The listing builds one solid part. Answer for the finished solid, in the listing's coordinates (mm). Face numbers are marked on the shaded views. A direction names the side the tool comes from. Coordinates: 2 decimals unless noted, no trailing zeros. Order: outer loops, then holes, each group sorted by start corner. A loop starts at its lowest first (then second) coordinate and runs counter-clockwise, first axis right, second up. Notation, with made-up numbers: (-22.5, 4) -> (27.5, 4) arc R23 cw to (27.5, 22) -> close; hole circle Ø5 at (-15.5, 29). An arc over 180 degrees is marked (long way). Answer in a Markdown table with one row per item. Add a question column.
```python
from build123d import *

# Parameters (mm, degrees)
SKETCH_W     = 25
SKETCH_H     = 32
PAD_DEPTH    = 2
SKETCH001_W  = 22
SKETCH001_H  = 30
PAD001_DEPTH = 16.200001
SKETCH002_W  = 17.2
SKETCH002_H  = 24.2
POCKET_DEPTH = 16
SKETCH003_W  = 1
SKETCH003_H  = 8
PAD002_DEPTH = 10
PAD003_DEPTH = 8.5
FILLET_R     = 1
FILLET001_R  = 0.75
FILLET002_R  = 1
FILLET003_R  = 0.75


with BuildPart() as part:
    # Sketch → Pad (new body)
    with BuildSketch(Plane.XY):
        Rectangle(SKETCH_W, SKETCH_H)
    extrude(amount=PAD_DEPTH)

    # Sketch001 → Pad001 (new body)
    with BuildSketch(Plane(origin=(0, 0, 0), x_dir=(1, 0, 0), z_dir=(0, 0, -1))):
        Rectangle(SKETCH001_W, SKETCH001_H)
    extrude(amount=PAD001_DEPTH)

    # Sketch002 → Pocket (cut)
    with BuildSketch(Plane.XY.offset(2)):
        Rectangle(SKETCH002_W, SKETCH002_H)
    extrude(amount=-POCKET_DEPTH, mode=Mode.SUBTRACT)

    # Sketch003 → Pad002 (new body)
    with BuildSketch(Plane.XY.offset(-14)):
        with Locations((-0.5, 0)):
            Rectangle(SKETCH003_W, SKETCH003_H)
    extrude(amount=PAD002_DEPTH)

    # Sketch004 → Pad003 (new body, symmetric)
    with BuildSketch(Plane.YZ):
        with BuildLine():
            Line((-1.421224, -2.628412), (0.611463, -8.650596))
            ThreePointArc((0.611463, -8.650596), (2.512397, -9.59211), (3.453911, -7.691175))
            Line((3.453911, -7.691175), (1.421224, -1.668991))
            Line((1.421224, -1.668991), (11.362733, 1.686598))
            ThreePointArc((11.362733, 1.686598), (8.973628, 5.807128), (5.169008, 8.672693))
            ThreePointArc((-10.669687, 3.326607), (-1.936582, 3.588753), (5.169008, 8.672693))
            ThreePointArc((-10.669687, 3.326607), (-11.959462, -1.258485), (-11.362733, -5.984001))
            Line((-1.421224, -2.628412), (-11.362733, -5.984001))
        make_face()
    extrude(amount=PAD003_DEPTH, both=True)

    # Fillet
    fillet_edges = [part.edges().sort_by_distance(p)[0] for p in [
        (-12.5, -16, 1),
        (12.5, -16, 1),
        (12.5, 16, 1),
        (-12.5, 16, 1),
    ]]
    fillet(fillet_edges, radius=FILLET_R)

    # Fillet001
    fillet001_edges = [part.edges().sort_by_distance(p)[0] for p in [
        (0, -16, 2),
    ]]
    fillet(fillet001_edges, radius=FILLET001_R)

    # Fillet002
    fillet002_edges = [part.edges().sort_by_distance(p)[0] for p in [
        (0, -10.669687, 3.326607),
        (0, 5.169008, 8.672693),
    ]]
    fillet(fillet002_edges, radius=FILLET002_R)

    # Fillet003
    fillet003_edges = [part.edges().sort_by_distance(p)[0] for p in [
        (8.5, -1.936582, 3.588753),
        (-8.5, -1.936582, 3.588753),
    ]]
    fillet(fillet003_edges, radius=FILLET003_R)


solid = part.part
```
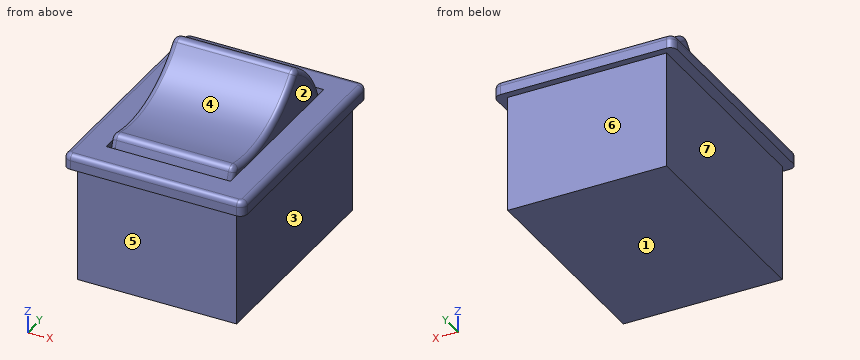
Q1. For the marked faces 1, 2 and 3, determine the directions among +Z, -Z, +X, -X, +Y, -Y from which every point of the face is accessible in a straight line to the end or side of a thin tool.
Q2. A cutting plane is placed at C-C (z = -3.5). State how many separate pieces and enclosed holes the cut face has, then the cut area to 3 significant figures.
Q3. Given pin 1 (3 mm diameter, centred on y = 12, z = -6.5, fed in from -X); pin 2 (6 mm diameter, centred on y = -4.5, z = -9.5, fed in from +X); pin 3 (1 mm diameter, centred on x = -4, z = -13, fed in from -Y); pin 4 (8 mm diameter, centred on x = -8.5, z = -1.5, fed in from +Y), each flat-ended and moving along its own axis, determine where each tip first touches the part or whether it passes through.
Q4. Straight lines are drawn through the part: line 1 (X direction, y = -3, z = -7.5); line 2 (X direction, y = -12, z = -9); line 3 (Z direction, x = -5.25, y = -2). For each, find the intervals that lie inside material, in ascending order.
Q5. Determine the mould class of the marked faces 4, 5, 6 and 7 for opening direction Y: +Y half, -Y half, draft (parallel to the pull), parting line (faces both ways), or undercut.
Q6. A cutting plane is placed at A-A (z = -10.75). Determine the outline of the cut face in (x, y), then the cut area to 3 significant figures.
Q7. A cutting plane is placed at B-B (x = 10.25). Determine the outline of the cut face in (y, z).
Returned:
| question | item | result |
|---|---|---|
| 1 | face 1 | -Z, +X, -X, +Y, -Y |
| 1 | face 2 | +Z |
| 1 | face 3 | -Z, +X, +Y, -Y |
| 2 | separate pieces | 3 |
| 2 | enclosed holes | 1 |
| 2 | area | 432 mm² |
| 3 | pin 1 | stops at x = -11 |
| 3 | pin 2 | stops at x = 11 |
| 3 | pin 3 | stops at y = -15 |
| 3 | pin 4 | stops at y = 16 |
| 4 | line 1 | x = -11 to -8.6, -1 to 0, 8.6 to 11 |
| 4 | line 2 | x = -11 to -8.6, 8.6 to 11 |
| 4 | line 3 | z = -16.2 to -14, -2.82 to 3.57 |
| 5 | face 4 | undercut |
| 5 | face 5 | -Y half |
| 5 | face 6 | +Y half |
| 5 | face 7 | draft |
| 6 | outline | (-11, -15) -> (11, -15) -> (11, 15) -> (-11, 15) -> close; (-1, -4) -> (0, -4) -> (0, 4) -> (-1, 4) -> close; hole (-8.6, -12.1) -> (8.6, -12.1) -> (8.6, 12.1) -> (-8.6, 12.1) -> close |
| 6 | area | 252 mm² |
| 7 | outline | (-16, 0) -> (-15, 0) -> (-15, -16.2) -> (15, -16.2) -> (15, 0) -> (16, 0) -> (16, 1.25) arc R0.75 ccw to (15.25, 2) -> (-15.25, 2) arc R0.75 ccw to (-16, 1.25) -> close |
